from build123d import *

# Parameters (mm, degrees)
SKETCH_1_R      = 2
SKETCH_1_R_2    = 1.5
EXTRUDE_1_DEPTH = 2
FILLET_1_R      = 3
FILLET_2_R      = 4
FILLET_3_R      = 1
SKETCH_2_R      = 3
SKETCH_2_R_2    = 2
EXTRUDE_2_DEPTH = 0.75


with BuildPart() as part:
    # 草图1 → 凸台-拉伸1 (new body)
    with BuildSketch(Plane(origin=(0, 0, -37.252464054), x_dir=(0.999999999, -4.5024e-05, 0), z_dir=(0, 0, 1))):
        Polygon((-10.738945167, 10.350396652), (-14.113721921, 22.945234964), (-20.875202705, 21.133501648), (-17.261865242, 7.64834265), (-12.97599562, 0.225770523), (-9.524857048, 0.225770523), (-11.024974023, 2.823779195), (-9.229747105, 2.823860024), (-7.811543717, 5.280515782), align=None)
        with Locations((-16.588595655, 18.658627914)):
            Circle(SKETCH_1_R, mode=Mode.SUBTRACT)
        with Locations((-14.000405204, 8.999369651)):
            Circle(SKETCH_1_R_2, mode=Mode.SUBTRACT)
    extrude(amount=EXTRUDE_1_DEPTH)

    # 圆角1
    fillet_1_edges = [part.edges().sort_by_distance(p)[0] for p in [
        (-10.738479137, 10.350880155, -36.252464054),
        (-14.112688814, 22.945870401, -36.252464054),
        (-20.874251163, 21.134441518, -36.252464054),
        (-17.261520863, 7.649119845, -36.252464054),
    ]]
    fillet(fillet_1_edges, radius=FILLET_1_R)

    # 圆角2
    fillet_2_edges = [part.edges().sort_by_distance(p)[0] for p in [
        (-7.811305958, 5.280867486, -36.252464054),
    ]]
    fillet(fillet_2_edges, radius=FILLET_2_R)

    # 圆角3
    fillet_3_edges = [part.edges().sort_by_distance(p)[0] for p in [
        (-12.975985442, 0.226354757, -36.252464054),
    ]]
    fillet(fillet_3_edges, radius=FILLET_3_R)

    # 草图2 → 凸台-拉伸2 (add)
    with BuildSketch(Plane(origin=(-0.25104956, -0.068074204, -37.252464054), x_dir=(1, 0, 0), z_dir=(0, 0, 1))):
        with Locations((-16.336705988, 18.727448988)):
            Circle(SKETCH_2_R)
        with Locations((-16.336705988, 18.727448988)):
            Circle(SKETCH_2_R_2, mode=Mode.SUBTRACT)
    extrude(amount=-EXTRUDE_2_DEPTH)


solid = part.part
Check sheet for the modelled part. Datum: model origin and axes. Units: mm. A direction names the side the tool comes from. Round coordinates to 2 decimals unless told otherwise and drop trailing zeros. Write each loop counter-clockwise with the first axis right and the second up, starting at its lowest first coordinate (ties: lowest second). Pieces come first, ordered by that corner, then holes. Notation, with made-up numbers: (19, 26.5) - (78, 26.5) arc R10 ccw to (78, 31.5) - close; hole circle Ø3 at (-17.5, -37.75). An arc over 180 degrees is marked (long way). Return JSON: item names as keys, results as strings.
Q1. Access from +Z, -Z, +X, -X, +Y, -Y to the whole of each face (thin tool, end or side, straight path). Record for faces 4 (the cylindrical face through (-19.585, 18.791, -37.622)), 5 (the flat face through (-12.071, 15.325, -36.266)), 6 (the flat face through (-10, 2.824, -36)).
Returned:
{"face 4": "-Z", "face 5": "+Z, -Z, +X, +Y", "face 6": "+Z, -Z, +X"}
Q2. Cross-section at B-B (z = -37.5). Record the boundary of the cut face in (x, y).
Returned:
{"outline": "circle Ø6 at (-16.59, 18.66); hole circle Ø4 at (-16.59, 18.66)"}
Q3. Cross-section at A-A (x = -14). Record the boundary of the cut face in (y, z).
Returned:
{"outline": "(2, -37.25) - (7.5, -37.25) - (7.5, -35.25) - (2, -35.25) - close; (10.5, -37.25) - (17.14, -37.25) - (17.14, -38) - (20.18, -38) - (20.18, -37.25) - (21.27, -37.25) - (21.27, -35.25) - (10.5, -35.25) - close"}
Q4. Cross-section at C-C (y = 4). Record the boundary of the cut face in (x, z).
Returned:
{"outline": "(-15.15, -37.25) - (-8.64, -37.25) - (-8.64, -35.25) - (-15.15, -35.25) - close"}
Q5. Draft check along Y on faces 1 (the flat face through (-10.264, 1.507, -36.266)), 2 (the flat face through (-19, 19, -38.002)), 3 (the cylindrical face through (-8.43, 5.31, -36.24)). Enter one of: released by +Y, released by -Y, zero draft, split by the parting line, or undercut.
Returned:
{"face 1": "undercut", "face 2": "zero draft", "face 3": "split by the parting line"}
Q6. Cross-section at D-D (x = -8.75). Record the boundary of the cut face in (y, z).
Returned:
{"outline": "(3.71, -37.25) - (6.85, -37.25) - (6.85, -35.25) - (3.71, -35.25) - close"}
Q7. Scan lines: L1, parallel to Z at x = -19, y = 16.5; L2, parallel to X at y = 17.25, z = -37.4; L3, parallel to Y at x = -14, z = -35.75. Record each from-to range of solid material in increasing order. Write a range as from..to.
Returned:
{"L1": "z = -37.25..-35.25", "L2": "x = -19.24..-18.01, -15.17..-13.94", "L3": "y = 2..7.5, 10.5..21.27"}
Q8. Depth check by flat-ended pin: P1, Ø1.5, axis at x = -14.5, z = -36, coming from the -Y side. Enter the tip coordinate at first touch or a pass-through.
Returned:
{"P1": "stops at y = 1.57"}
